For this review, take the finished solid that the model builds, in its own axes (mm). Face numbers are marked on the shaded views. A direction names the side the tool comes from. Round coordinates to 2 decimals unless told otherwise and drop trailing zeros. Order: outer loops, then holes, each group sorted by start corner. A loop starts at its lowest first (then second) coordinate and runs counter-clockwise, first axis right, second up. Notation, with made-up numbers: (58.5, 83.5) -> (104.5, 83.5) arc R25 ccw to (104.5, 102.5) -> close; hole circle Ø1 at (59, -11.75). An arc over 180 degrees is marked (long way). Answer in a Markdown table with one row per item.
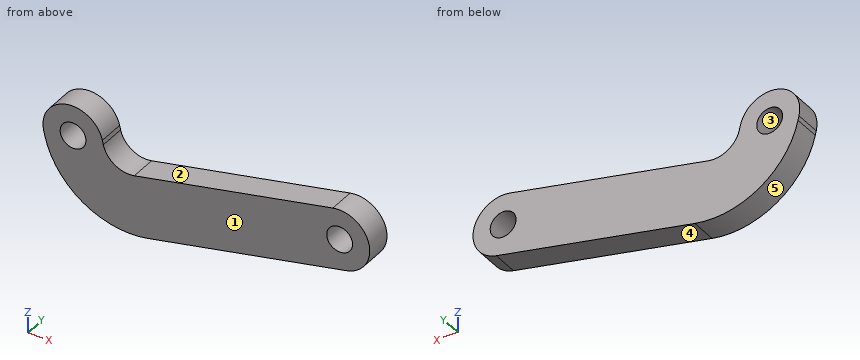
```python
from build123d import *

# Parameters (mm, degrees)
SKETCH1_R           = 1.5
BOSS_EXTRUDE1_DEPTH = 3


with BuildPart() as part:
    # Sketch1 → Boss-Extrude1 (new body)
    with BuildSketch(Plane(origin=(0, 0, 0), x_dir=(1, 0, 0), z_dir=(0, 1, 0))):
        with BuildLine():
            Line((3.409602648, -0.790322581), (3.522505874, -0.303236488))
            ThreePointArc((3.522505874, -0.303236488), (4.857498975, 1.564883251), (7.122441784, 1.941860713))
            Line((7.122441784, 1.941860713), (30.209677419, -3.409602648))
            ThreePointArc((30.209677419, -3.409602648), (34.409602648, -0.790322581), (31.790322581, 3.409602648))
            Line((31.790322581, 3.409602648), (8.703086946, 8.761066009))
            ThreePointArc((8.703086946, 8.761066009), (1.153277579, 7.504474471), (-3.296699422, 1.277408673))
            Line((-3.296699422, 1.277408673), (-3.409602648, 0.790322581))
            ThreePointArc((-3.409602648, 0.790322581), (-0.790322581, -3.409602648), (3.409602648, -0.790322581))
        make_face()
        Circle(SKETCH1_R, mode=Mode.SUBTRACT)
        with Locations((31, 0)):
            Circle(SKETCH1_R, mode=Mode.SUBTRACT)
    extrude(amount=BOSS_EXTRUDE1_DEPTH)


solid = part.part
```
Q1. To check wall thickness, follow probe 1 along Z at (x, y) = (0, 1.45); probe 2 along Z at (x, y) = (31, 0.6); probe 3 along Z at (x, y) = (27, 0.85). State the ranges of each line that lie inside material, in increasing order.
Answer key:
| item | result |
|---|---|
| probe 1 | z = -6.67 to -1.5, 1.5 to 3.5 |
| probe 2 | z = -3.59 to -1.5, 1.5 to 3.5 |
| probe 3 | z = -4.52 to 2.67 |
Q2. Take a section at A-A, the plane y = 0.7. Write out the cut boundary in (x, z), then the cut area to 3 significant figures.
Answer key:
| item | result |
|---|---|
| outline | (-3.41, -0.79) -> (-3.3, -1.28) arc R10 ccw to (8.7, -8.76) -> (31.79, -3.41) arc R3.5 ccw to (30.21, 3.41) -> (7.12, -1.94) arc R3 cw to (3.52, 0.3) -> (3.41, 0.79) arc R3.5 ccw to start; hole circle Ø3 at (0, 0); hole circle Ø3 at (31, 0) |
| area | 265 mm^2 |
Q3. Take a section at D-D, the plane x = 4.5. Write out the cut boundary in (y, z).
Answer key:
| item | result |
|---|---|
| outline | (0, -8.83) -> (3, -8.83) -> (3, -1.3) -> (0, -1.3) -> close |
Q4. Tool access review of the marked faces 1 and 2: name each direction out of +Z, -Z, +X, -X, +Y, -Y from which nothing blocks a thin tool from reaching the whole face with its end or side.
Answer key:
| item | result |
|---|---|
| face 1 | +Z, -Z, +X, -X, -Y |
| face 2 | +Z, +Y, -Y |
Q5. The part is to be moulded in two halves that separate along X. For the marked faces 3, 4 and 5, say which applies: +X half, -X half, draft (parallel to the pull), parting line (faces both ways), or undercut.
Answer key:
| item | result |
|---|---|
| face 3 | undercut |
| face 4 | +X half |
| face 5 | parting line |
Q6. Take a section at B-B, the plane x = 0. Write out the cut boundary in (y, z).
Answer key:
| item | result |
|---|---|
| outline | (0, -6.67) -> (3, -6.67) -> (3, -1.5) -> (0, -1.5) -> close; (0, 1.5) -> (3, 1.5) -> (3, 3.5) -> (0, 3.5) -> close |
Q7. Take a section at C-C, the plane z = -7. Write out the cut boundary in (x, y), then the cut area to 3 significant figures.
Answer key:
| item | result |
|---|---|
| outline | (0.42, 0) -> (16.3, 0) -> (16.3, 3) -> (0.42, 3) -> close |
| area | 47.6 mm^2 |
